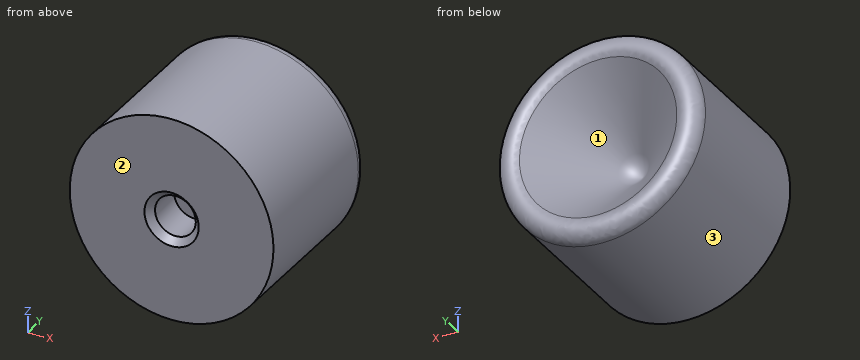
```python
from build123d import *

# Parameters (mm, degrees)
FILLET1_R     = 2
CHAMFER1_SIZE = 1


with BuildPart() as part:
    # Sketch1 → Revolve1 (revolve)
    with BuildSketch(Plane(origin=(0, 0, 0), x_dir=(0, 0, -1), z_dir=(1, 0, 0))):
        Polygon((0, 0), (15, 15), (15, -12), (3, -12), (3, -6), (0, -6), align=None)
    revolve(axis=Axis((0, -6, 0), (0, 1, 0)))

    # Fillet1
    fillet1_edges = [part.edges().sort_by_distance(p)[0] for p in [
        (0, 15, 15),
    ]]
    fillet(fillet1_edges, radius=FILLET1_R)

    # Chamfer1
    chamfer1_edges = [part.edges().sort_by_distance(p)[0] for p in [
        (0, -12, 3),
    ]]
    chamfer(chamfer1_edges, length=CHAMFER1_SIZE)


solid = part.part
```
Work out the finished part from the listing and answer in its coordinate system (mm). Face numbers are marked on the shaded views. Round coordinates to 2 decimals unless told otherwise and drop trailing zeros. Write each loop counter-clockwise with the first axis right and the second up, starting at its lowest first coordinate (ties: lowest second). Pieces come first, ordered by that corner, then holes. Notation, with made-up numbers: (-15, 41.5) - (44, 41.5) arc R22 ccw to (44, 51.5) - close; hole circle Ø2 at (9, -20). An arc over 180 degrees is marked (long way). Return JSON: item names as keys, results as strings. Group by question number.
Q1. The part is cut by section C-C on y = 8.5. Write down the section's boundary in (x, z), then the cut area to 3 significant figures.
Q2. The part is cut by section A-A on y = 4.5. Write down the section's boundary in (x, z), then the cut area to 3 significant figures.
Q3. Each of these flat-tipped pins is pushed along its axis until it touches: pin 1 Ø8 at (x, y) = (11.5, 6.5) entering from -Z; pin 2 Ø4 at (y, z) = (-4.5, 4.5) entering from -X; pin 3 Ø2 at (x, y) = (1.5, -2.5) entering from -Z. Where does it stop, or does it pass through?
Q4. The part is cut by section B-B on y = -0.5. Write down the section's boundary in (x, z).
Q5. Find the intervals of material crossed by L1, parallel to Z at x = 0, y = -9.2; L2, parallel to Z at x = -7, y = 10.75, in increasing order.
Q6. The mould has two halves that part along X. Classify the marked faces 1, 2 and 3: released by +X, released by -X, zero draft, split by the parting line, or undercut.
Solved:
{
 "1": {"outline": "circle Ø30 at (0, 0); hole circle Ø17 at (0, 0)", "area": "480 mm²"},
 "2": {"outline": "circle Ø30 at (0, 0); hole circle Ø9 at (0, 0)", "area": "643 mm²"},
 "3": {"pin 1": "z = -12.99", "pin 2": "x = -14.79", "pin 3": "z = -14.99"},
 "4": {"outline": "circle Ø30 at (0, 0)"},
 "5": {"L1": "-15 to -3, 3 to 15", "L2": "-13.17 to -8.16, 8.16 to 13.17"},
 "6": {"face 1": "undercut", "face 2": "zero draft", "face 3": "split by the parting line"}
}
